The figure shows three views and two pictorial views of one solid part (mm, origin at its lowest corner). Answer the questions. A direction names the side the tool comes from. Coordinates: 2 decimals unless noted, no trailing zeros. Write each loop counter-clockwise with the first axis right and the second up, starting at its lowest first coordinate (ties: lowest second). Pieces come first, ordered by that corner, then holes. Notation, with made-up numbers: (45, -23) - (102, -23) arc R11 ccw to (102, -2) - close; hole circle Ø10 at (-1, 41). An arc over 180 degrees is marked (long way). Use a Markdown table: item, result. Add a question column.
(1) The part is cut by section B-B, the plane y = 18.5. Give the vertices of the cut face in (x, z), then the cut area to 3 significant figures.
(2) The part is cut by section D-D, the plane z = 3.75. Give the vertices of the cut face in (x, y), then the cut area to 3 significant figures.
(3) For a pull along X with two mould halves and no side action, classify the marked faces 1, 2, 3 and 4 as released by +X, released by -X, zero draft, split by the parting line, or undercut.
(4) A tool of negligible diameter and unlimited length cuts with its end or side. For the marked faces 5, 6 and 7, from which of +Z, -Z, +X, -X, +Y, -Y can it reach the whole face along a straight path? Write none if from no direction.
(5) The part is cut by section C-C, the plane x = 9.25. Give the vertices of the cut face in (y, z), then the cut area to 3 significant figures.
(6) Find the intervals of material crossed by line 1 (X direction, y = 9.5, z = 1); line 2 (X direction, y = 14.75, z = 5.25), in increasing order. Write a range as from..to.
(7) Given pin 1 Ø0.9 at (y, z) = (19, 6.5) entering from -X; pin 2 Ø1 at (x, y) = (26, 19) entering from -Z; pin 3 Ø0.9 at (x, z) = (10.5, 7) entering from +Y, each flat-ended and moving along its own axis, determine where each tip first touches the part or whether it passes through.
(8) The part is cut by section A-A, the plane z = 6.75. Give the vertices of the cut face in (x, y).
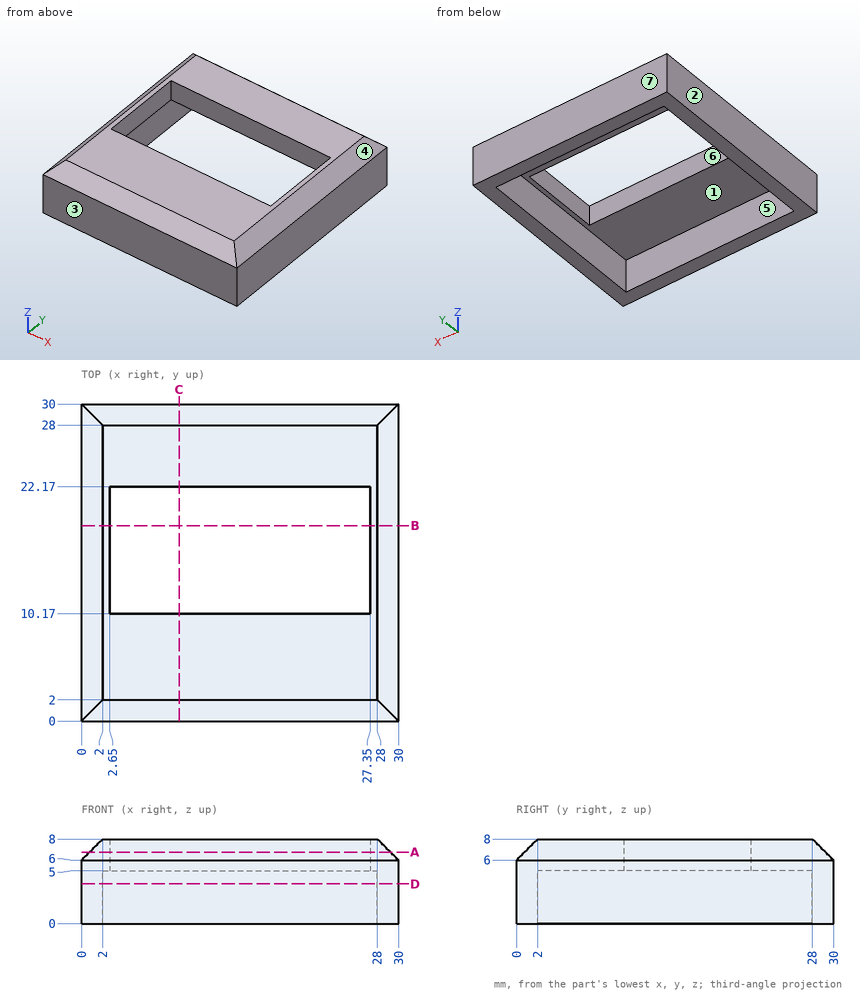
Model answer:
| question | item | result |
|---|---|---|
| 1 | outline | (0, 0) - (2, 0) - (2, 5) - (2.65, 5) - (2.65, 8) - (2, 8) - (0, 6) - close; (27.35, 5) - (28, 5) - (28, 0) - (30, 0) - (30, 6) - (28, 8) - (27.35, 8) - close |
| 1 | area | 31.9 mm^2 |
| 2 | outline | (0, 0) - (30, 0) - (30, 30) - (0, 30) - close; hole (2, 2) - (28, 2) - (28, 28) - (2, 28) - close |
| 2 | area | 224 mm^2 |
| 3 | face 1 | undercut |
| 3 | face 2 | released by -X |
| 3 | face 3 | zero draft |
| 3 | face 4 | released by +X |
| 4 | face 5 | -Z |
| 4 | face 6 | +Z, -Z |
| 4 | face 7 | +Z, -Z, +X, -X, +Y |
| 5 | outline | (0, 0) - (2, 0) - (2, 5) - (10.17, 5) - (10.17, 8) - (2, 8) - (0, 6) - close; (22.17, 5) - (28, 5) - (28, 0) - (30, 0) - (30, 6) - (28, 8) - (22.17, 8) - close |
| 5 | area | 70.0 mm^2 |
| 6 | line 1 | 0..2, 28..30 |
| 6 | line 2 | 0..2.65, 27.35..30 |
| 7 | pin 1 | x = 0.05 |
| 7 | pin 2 | through |
| 7 | pin 3 | y = 29.45 |
| 8 | outline | (0.75, 0.75) - (29.25, 0.75) - (29.25, 29.25) - (0.75, 29.25) - close; hole (2.65, 10.17) - (27.35, 10.17) - (27.35, 22.17) - (2.65, 22.17) - close |
